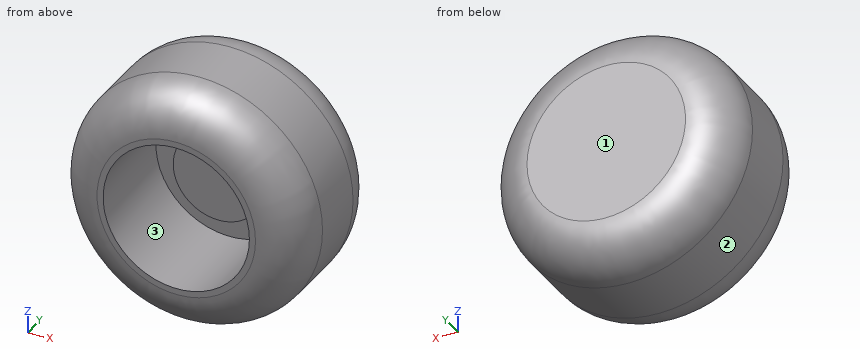
from build123d import *

# Parameters (mm, degrees)
F0_R     = 14.331374
F1_DEPTH = 16.764
F2_R     = 5.08
F3_R     = 5.08
F4_R     = 8.539137
F5_DEPTH = 11.43
F6_R     = 5.252723
F7_DEPTH = 2.3622


with BuildPart() as f1:
    # F0 (on Front) → F1 (new body)
    with BuildSketch(Plane.XZ):
        Circle(F0_R)
    extrude(amount=F1_DEPTH)

    # F2
    f2_edges = [f1.edges().sort_by_distance(p)[0] for p in [
        (-14.331374, -16.764, 0),
    ]]
    fillet(f2_edges, radius=F2_R)

    # F3
    f3_edges = [f1.edges().sort_by_distance(p)[0] for p in [
        (-14.331374, 0, 0),
    ]]
    fillet(f3_edges, radius=F3_R)

    # F4 (on face) → F5 (cut)
    with BuildSketch(Plane.XZ.offset(16.764)):
        Circle(F4_R)
    extrude(amount=-F5_DEPTH, mode=Mode.SUBTRACT)

    # F6 (on face) → F7 (join)
    with BuildSketch(Plane.XZ.offset(5.334)):
        Circle(F6_R)
    extrude(amount=F7_DEPTH)


solid = f1.part
Design review of the part built by this model. Coordinates are the model's own, in mm. Face numbers are marked on the shaded views. Round coordinates to 2 decimals unless told otherwise and drop trailing zeros. Write each loop counter-clockwise with the first axis right and the second up, starting at its lowest first coordinate (ties: lowest second). Pieces come first, ordered by that corner, then holes.
Item 1: Consider section C-C on x = 0. Give the boundary of the cut face in (y, z), and give its area (3 significant figures).
Item 2: Consider section B-B on z = 0. Give the boundary of the cut face in (x, y).
Item 3: Wall thickness on L1, parallel to Z at x = 0, y = -11; L2, parallel to Z at x = -4.25, y = -7.25; L3, parallel to Y at x = 5.5, z = 5.25: over which ranges is each line inside the solid? List them lowest first.
Item 4: Consider section D-D on y = -9.5. Give the boundary of the cut face in (x, z), and give its area (3 significant figures).
Item 5: For pin 1 Ø10 at (x, z) = (0, 0) entering from -Y; pin 2 Ø5 at (y, z) = (-14.5, -0.5) entering from -X; pin 3 Ø4 at (x, y) = (3.5, -14.5) entering from -Z, all flat-tipped, find the tip position at first contact; note any pin that passes through.
Item 6: Draft analysis for pull direction Z (two halves, no side actions). For the marked faces 1, 2 and 3, state which applies: released by +Z, released by -Z, zero draft, split by the parting line, or undercut.
Item 7: Consider section A-A on y = -6.5. Give the boundary of the cut face in (x, z), and give its area (3 significant figures).
Check values:
1. outline: (-16.76, -9.25) arc R5.08 ccw to (-11.68, -14.33) - (-5.08, -14.33) arc R5.08 ccw to (0, -9.25) - (0, 9.25) arc R5.08 ccw to (-5.08, 14.33) - (-11.68, 14.33) arc R5.08 ccw to (-16.76, 9.25) - (-16.76, 8.54) - (-5.33, 8.54) - (-5.33, 5.25) - (-7.7, 5.25) - (-7.7, -5.25) - (-5.33, -5.25) - (-5.33, -8.54) - (-16.76, -8.54) - close
1. area: 288 mm2
2. outline: (-14.33, -11.68) arc R5.08 ccw to (-9.25, -16.76) - (-8.54, -16.76) - (-8.54, -5.33) - (-5.25, -5.33) - (-5.25, -7.7) - (5.25, -7.7) - (5.25, -5.33) - (8.54, -5.33) - (8.54, -16.76) - (9.25, -16.76) arc R5.08 ccw to (14.33, -11.68) - (14.33, -5.08) arc R5.08 ccw to (9.25, 0) - (-9.25, 0) arc R5.08 ccw to (-14.33, -5.08) - close
3. L1: z = -14.33 to -8.54, 8.54 to 14.33
3. L2: z = -13.69 to -7.41, -3.09 to 3.09, 7.41 to 13.69
3. L3: y = -5.33 to 0
4. outline: circle Ø28.66 at (0, 0); hole circle Ø17.08 at (0, 0)
4. area: 416 mm2
5. pin 1: stops at y = -7.7
5. pin 2: stops at x = -14.32
5. pin 3: stops at z = -14
6. face 1: zero draft
6. face 2: split by the parting line
6. face 3: undercut
7. outline: circle Ø28.66 at (0, 0); circle Ø10.51 at (0, 0); hole circle Ø17.08 at (0, 0)
7. area: 503 mm2
